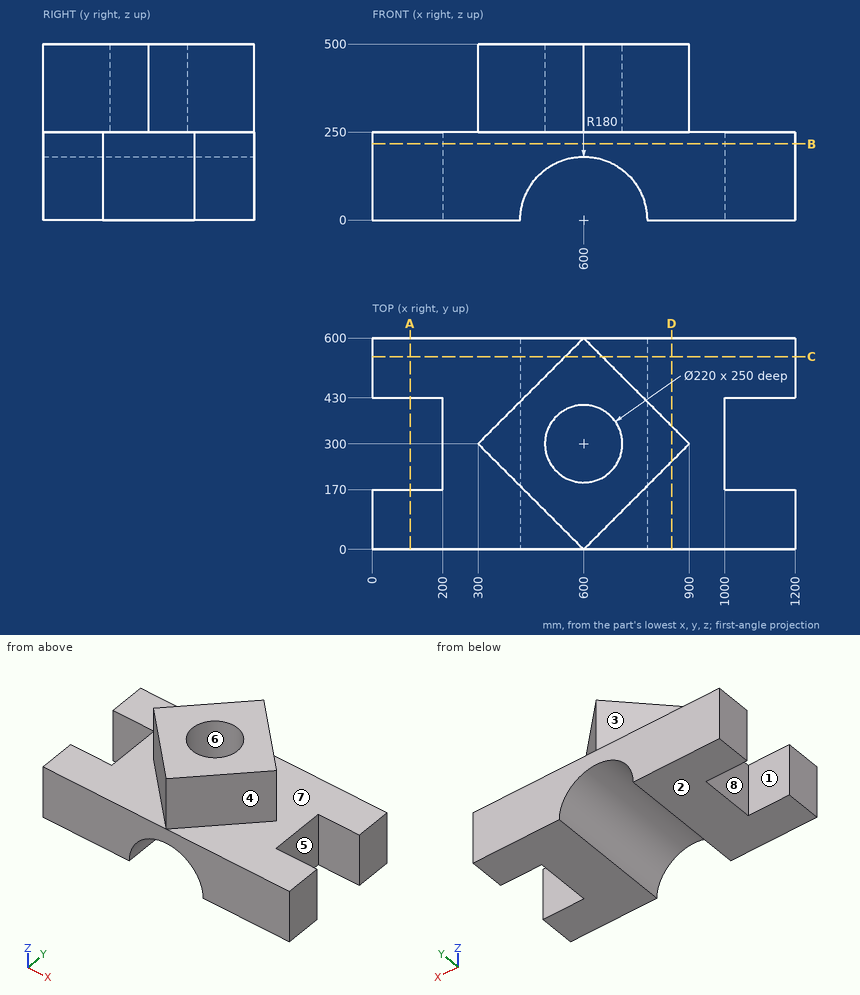
Here's the drawing with two shaded views (mm, measured from the low corner). I have some questions. A direction names the side the tool comes from. Coordinates: 2 decimals unless noted, no trailing zeros. Order: outer loops, then holes, each group sorted by start corner. A loop starts at its lowest first (then second) coordinate and runs counter-clockwise, first axis right, second up.
Q1. Suppose I cut it at C-C on y = 547.5. Please give me the cut outline in (x, z).
Q2. Thinking about a two-plate mould opening in Y: for the marked faces 1, 2 and 3, which applies, released by +Y, released by -Y, zero draft, split by the parting line, or undercut?
Q3. Which directions (+Z, -Z, +X, -X, +Y, -Y) give clear straight access to the entire face, cutting with the end or side of a thin tool? Please do the marked faces 4, 5, 6, 7 and 8.
Q4. Suppose I cut it at B-B on z = 216.5. Please give me the cut outline in (x, y).
Q5. Suppose I cut it at D-D on x = 850. Please give me the cut outline in (y, z), and give its area (3 significant figures).
Q6. Please list where these lines run through material, in increasing order: L1, parallel to Y at x = 600, z = 324; L2, parallel to Y at x = 652, z = 419; L3, parallel to Z at x = 119.5, y = 499.5.
Q7. Will these pins go through, and if not, where does the flat tip stop? pin 1 (2 mm diameter, centred on x = 513, z = 402, fed in from +Y); pin 2 (1 mm diameter, centred on y = 453, z = 330, fed in from +X); pin 3 (8 mm diameter, centred on x = 356.5, z = 418.5, fed in from +Y).
Q8. Suppose I cut it at A-A on x = 107. Please give me the cut outline in (y, z), and give its area (3 significant figures).
Answer:
1. outline: (0, 0) - (420, 0) arc R180 cw to (780, 0) - (1200, 0) - (1200, 250) - (652.5, 250) - (652.5, 500) - (547.5, 500) - (547.5, 250) - (0, 250) - close
2. face 1: undercut
2. face 2: zero draft
2. face 3: released by +Y
3. face 4: +Z, +X, -Y
3. face 5: +Z, -Z, +X
3. face 6: +Z
3. face 7: +Z, +X
3. face 8: +Z, -Z, -X
4. outline: (0, 0) - (1200, 0) - (1200, 170) - (1000, 170) - (1000, 430) - (1200, 430) - (1200, 600) - (0, 600) - (0, 430) - (200, 430) - (200, 170) - (0, 170) - close
5. outline: (0, 0) - (600, 0) - (600, 250) - (350, 250) - (350, 500) - (250, 500) - (250, 250) - (0, 250) - close
5. area: 175,000 mm2
6. L1: y = 0 to 190, 410 to 600
6. L2: y = 52 to 203.07, 396.93 to 548
6. L3: z = 0 to 250
7. pin 1: stops at y = 514
7. pin 2: stops at x = 747.5
7. pin 3: stops at y = 360.5
8. outline: (0, 0) - (170, 0) - (170, 250) - (0, 250) - close; (430, 0) - (600, 0) - (600, 250) - (430, 250) - close
8. area: 85,000 mm2
